```python
from build123d import *

# Parameters (mm, degrees)
BOSS_EXTRUDE1_DEPTH     = 300
SKETCH3_R               = 15.5
CUT_EXTRUDE1_DEPTH      = 23
CUT_EXTRUDE1_DEPTH_BACK = 23
SKETCH4_R               = 35
CUT_EXTRUDE3_DEPTH      = 300
SKETCH5_W               = 550.332786852
SKETCH5_H               = 261.274024582
CUT_EXTRUDE4_DEPTH      = 201.0000001


with BuildPart() as part:
    # Sketch1 → Boss-Extrude1 (new body)
    with BuildSketch(Plane(origin=(0, 0, 0), x_dir=(1, 0, 0), z_dir=(0, 1, 0))):
        with BuildLine():
            Line((-200, 1e-09), (200, 1e-09))
            add(Edge.make_bspline(
                [(-200, 1e-09), (0, -400.000000001), (200, 1e-09)],
                knots=[0.056028396, 0.056028396, 0.056028396, 0.943971604, 0.943971604, 0.943971604], degree=2))
        make_face()
    extrude(amount=BOSS_EXTRUDE1_DEPTH)

    # Sketch3 → Cut-Extrude1 (cut, two sides)
    with BuildSketch(Plane(origin=(0, 150, 0), x_dir=(1, 0, 0), z_dir=(0, 1, 0))) as cut_extrude1_sk:
        with Locations((0, -142.999999999)):
            Circle(SKETCH3_R)
    extrude(amount=CUT_EXTRUDE1_DEPTH, mode=Mode.SUBTRACT)
    extrude(cut_extrude1_sk.sketch, amount=-CUT_EXTRUDE1_DEPTH_BACK, mode=Mode.SUBTRACT)

    # Sketch4 → Cut-Extrude3 (cut)
    with BuildSketch(Plane(origin=(0, 173, 0), x_dir=(1, 0, 0), z_dir=(0, 1, 0))):
        with Locations((0, -142.999999999)):
            Circle(SKETCH4_R)
    cut_extrude3 = extrude(amount=CUT_EXTRUDE3_DEPTH, mode=Mode.SUBTRACT)

    # Mirror1: Cut-Extrude3 across plane
    add(cut_extrude3.mirror(Plane.ZX.offset(150)), mode=Mode.SUBTRACT)

    # Sketch5 → Cut-Extrude4 (cut, through all)
    with BuildSketch(Plane(origin=(0, 0, 0), x_dir=(-1, 0, 0), z_dir=(0, 0, -1))):
        with Locations((-5.361966922, 176.637012291)):
            Rectangle(SKETCH5_W, SKETCH5_H)
    extrude(amount=-CUT_EXTRUDE4_DEPTH, mode=Mode.SUBTRACT)


solid = part.part
```
Could you check a few things on this model? Use its own coordinates, in mm. Coordinates: 2 decimals unless noted, no trailing zeros. Answer as CSV lines item,"result". Start each with the question number.
1) For P1, Ø1, axis at y = 6, z = 20, coming from the +X side; P2, Ø6, axis at y = 32.5, z = 69, coming from the -X side; P3, Ø3, axis at y = 23, z = 168.5, coming from the +X side; P4, Ø8, axis at x = 153.5, z = 64, coming from the -Y side, each with a flat end and sliding along its axis, tell me the tip position at first contact or that it passes through.
2) We'd pull the mould along X, two halves only. Please class faces 1 (the cylindrical face through (-7.587, 23.322, 177.168)), 2 (the flat face through (1, 0, 81)): +X half, -X half, draft (parallel to the pull), parting line (faces both ways), or undercut.
3) Please list where these lines run through material, in increasing order: line 1 (Z direction, x = 0, y = 26); line 2 (X direction, y = 15, z = 171.5); line 3 (Z direction, x = -24, y = 24.5). Write a range as from..to.
Data:
1,P1,"stops at x = 190"
1,P2,"stops at x = -163.71"
1,P3,"stops at x = 81.24"
1,P4,"stops at y = 0"
2,face 1,"undercut"
2,face 2,"draft"
3,line 1,"z = 0..108, 178..200"
3,line 2,"x = -75.5..-20.32, 20.32..75.5"
3,line 3,"z = 0..117.52, 168.48..197.12"
